For this review, use the dimensioned drawing (mm, ordinates from the lowest corner) and the shaded views. A direction names the side the tool comes from. Give positions to 0.01 mm unless a question says otherwise; leave off trailing zeros. Order: outer loops, then holes, each group sorted by start corner. A loop starts at its lowest first (then second) coordinate and runs counter-clockwise, first axis right, second up.
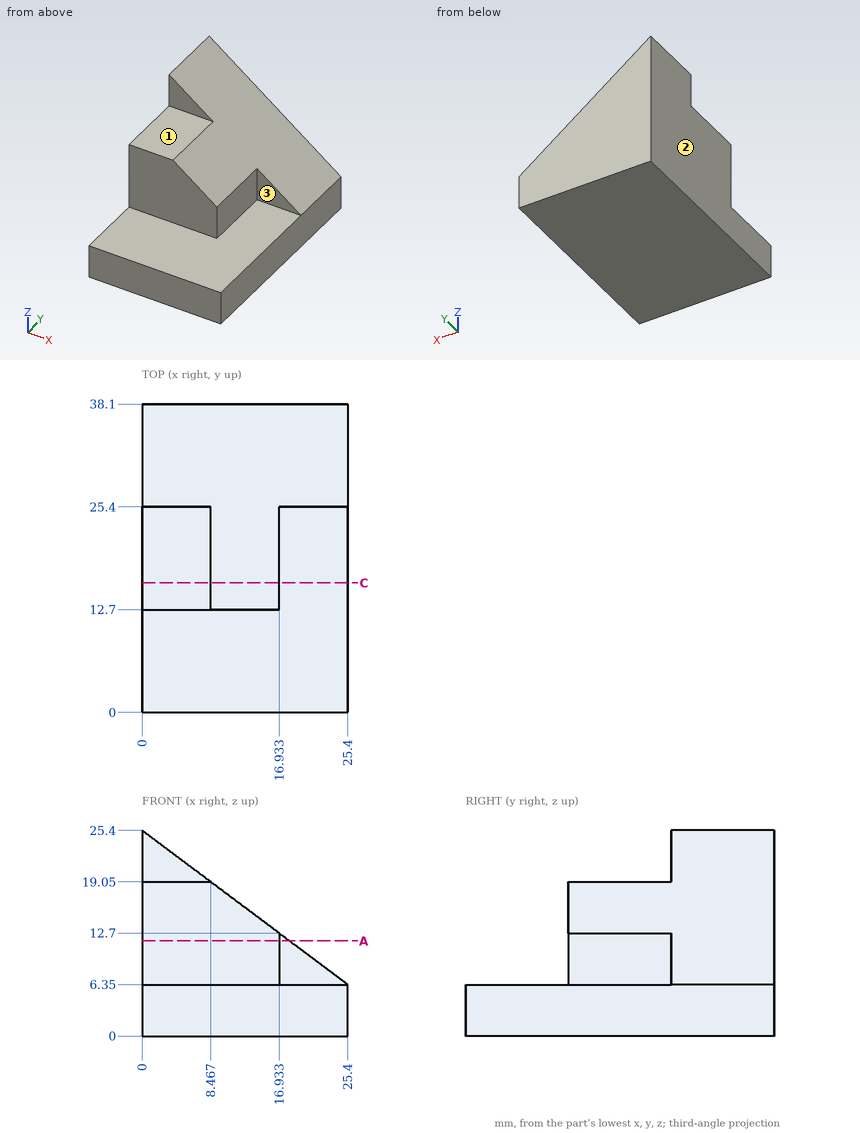
1. Take a section at A-A (z = 11.75). Write out the cut boundary in (x, y), and give its area (3 significant figures).
2. To check wall thickness, follow line 1 (Z direction, x = 6.5, y = 12); line 2 (Y direction, x = 3.25, z = 21); line 3 (Y direction, x = 3, z = 9). State the ranges of each line that lie inside material, in increasing order.
3. Take a section at C-C (y = 16). Write out the cut boundary in (x, z).
4. For the marked faces 1, 2 and 3, list the 3-axis set-ups (+Z, -Z, +X, -X, +Y, -Y) from which the entire face can be reached by the end or side of a thin tool; tool diameter is ignored.
5. Insertion check: pin 1 (10 mm diameter, centred on x = 11.5, z = 20.5, fed in from -Y); pin 2 (7.5 mm diameter, centred on x = 16.5, y = 16.5, fed in from +Z); pin 3 (3 mm diameter, centred on x = 3.5, z = 22.5, fed in from -Y); pin 4 (6 mm diameter, centred on y = 7, z = 20.5, fed in from -X). Each pin has a flat end and moves straight along its axis. Give the tip position at first contact, or say it passes through.
Answer:
1. outline: (0, 12.7) - (16.93, 12.7) - (16.93, 25.4) - (18.2, 25.4) - (18.2, 38.1) - (0, 38.1) - close
1. area: 446 mm2
2. line 1: z = 0 to 6.35
2. line 2: y = 25.4 to 38.1
2. line 3: y = 12.7 to 38.1
3. outline: (0, 0) - (25.4, 0) - (25.4, 6.35) - (16.93, 6.35) - (16.93, 12.7) - (8.47, 19.05) - (0, 19.05) - close
4. face 1: +Z, +X, -X, -Y
4. face 2: +Z, -Z, -X, +Y, -Y
4. face 3: +Z, +X, -Y
5. pin 1: stops at y = 12.7
5. pin 2: stops at z = 15.84
5. pin 3: stops at y = 25.4
5. pin 4: passes through
